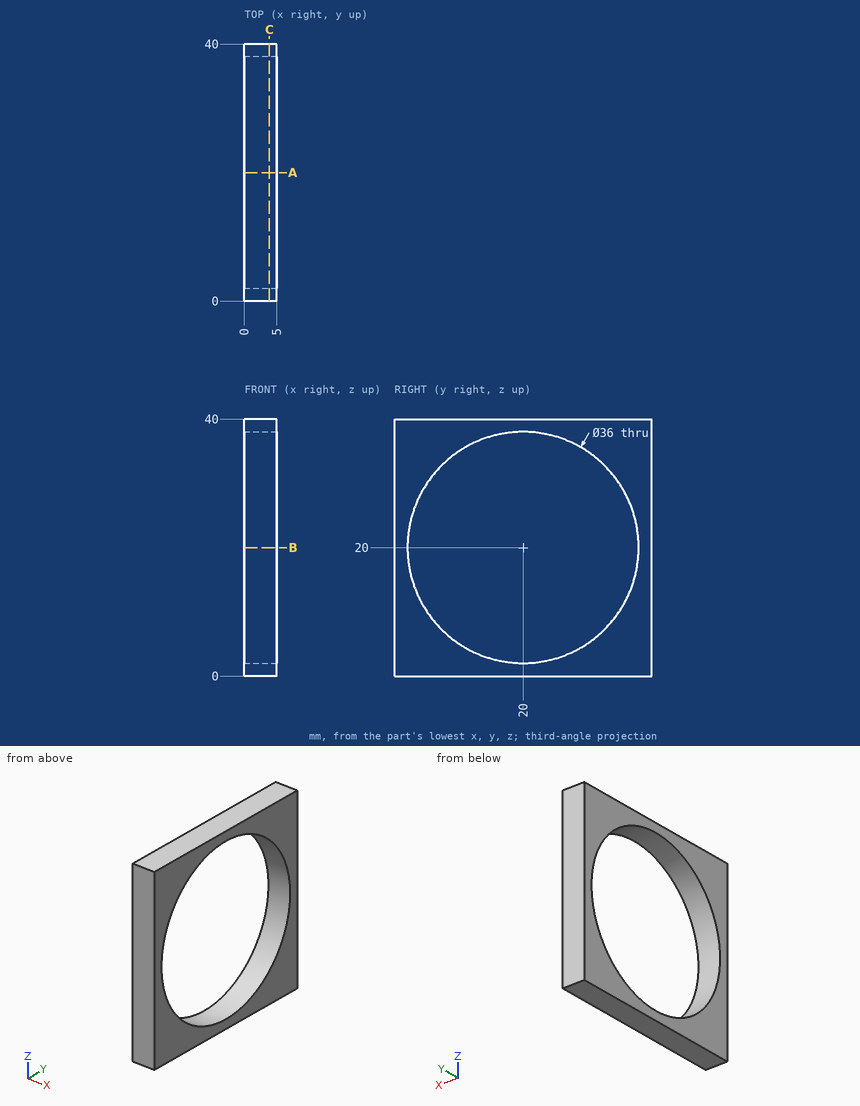
Check sheet for the drawn part. Datum: minimum x, y, z corner. Units: mm. Give positions to 0.01 mm unless a question says otherwise; leave off trailing zeros. Order: outer loops, then holes, each group sorted by start corner. A loop starts at its lowest first (then second) coordinate and runs counter-clockwise, first axis right, second up. Notation, with made-up numbers: (53.5, 4) - (65.5, 4) arc R26 cw to (65.5, 22) - close; hole circle Ø9 at (57.25, 27). An arc over 180 degrees is marked (long way). Answer in a Markdown table with one row per item. Add a question column.
Q1. Material ranges on probe 1 along Z at (x, y) = (2.2, 20); probe 2 along Z at (x, y) = (3.55, 23); probe 3 along Y at (x, z) = (4.55, 21), recorded low to high. Write a range as from..to.
Q2. Cross-section at C-C, the plane x = 3.9. Enter the section's corners in (y, z).
Q3. Gauge pin test, flat end, axial feed: pin 1 (8 mm diameter, centred on y = 22, z = 4.5, fed in from -X). Record the tip position at first contact, or that the pin passes through.
Q4. Cross-section at A-A, the plane y = 20. Enter the section's corners in (x, z).
Check values:
| question | item | result |
|---|---|---|
| 1 | probe 1 | z = 0..2, 38..40 |
| 1 | probe 2 | z = 0..2.25, 37.75..40 |
| 1 | probe 3 | y = 0..2.03, 37.97..40 |
| 2 | outline | (0, 0) - (40, 0) - (40, 40) - (0, 40) - close; hole circle Ø36 at (20, 20) |
| 3 | pin 1 | stops at x = 0 |
| 4 | outline | (0, 0) - (5, 0) - (5, 2) - (0, 2) - close; (0, 38) - (5, 38) - (5, 40) - (0, 40) - close |
